from build123d import *

# Parameters (mm, degrees)
SKETCH2_W           = 8.5
SKETCH2_H           = 6
BOSS_EXTRUDE1_DEPTH = 6
SKETCH3_W           = 6
SKETCH3_H           = 12
CUT_EXTRUDE1_DEPTH  = 6


with BuildPart() as part:
    # Sketch2 → Boss-Extrude1 (new body)
    with BuildSketch(Plane.XY):
        with Locations((-58.25, 3)):
            Rectangle(SKETCH2_W, SKETCH2_H)
        Polygon((-68.5, 72), (-68.5, 0), (-62.5, 0), (-62.5, 6), (-54, 6), (-42, 6), (-42, 0), (-30, 0), (-30, 6), (-18, 6), (-18, 0), (-6, 0), (-6, 6), (6, 6), (6, 0), (18, 0), (18, 6), (30, 6), (30, 0), (42, 0), (42, 6), (54, 6), (54, 0), (68.5, 0), (68.5, 72), (54, 72), (54, 66), (42, 66), (42, 72), (30, 72), (30, 66), (18, 66), (18, 72), (6, 72), (6, 66), (-6, 66), (-6, 72), (-18, 72), (-18, 66), (-30, 66), (-30, 72), (-42, 72), (-42, 66), (-54, 66), (-54, 72), align=None)
    extrude(amount=BOSS_EXTRUDE1_DEPTH)

    # Sketch3 → Cut-Extrude1 (cut)
    with BuildSketch(Plane.XY.offset(6)):
        with Locations((-65.5, 60)):
            Rectangle(SKETCH3_W, SKETCH3_H)
        with Locations((-65.5, 12)):
            Rectangle(SKETCH3_W, SKETCH3_H)
        with Locations((65.5, 36)):
            Rectangle(SKETCH3_W, SKETCH3_H)
        with Locations((65.5, 12)):
            Rectangle(SKETCH3_W, SKETCH3_H)
        with Locations((-65.5, 36)):
            Rectangle(SKETCH3_W, SKETCH3_H)
        with Locations((65.5, 60)):
            Rectangle(SKETCH3_W, SKETCH3_H)
    extrude(amount=-CUT_EXTRUDE1_DEPTH, mode=Mode.SUBTRACT)


solid = part.part
The listing builds one solid part. Answer for the finished solid, in the listing's coordinates (mm). A direction names the side the tool comes from. Give positions to 0.01 mm unless a question says otherwise; leave off trailing zeros. Write each loop counter-clockwise with the first axis right and the second up, starting at its lowest first coordinate (ties: lowest second). Pieces come first, ordered by that corner, then holes.
Item 1: Determine the mould class of faces 5 (the flat face through (-54, 3, 3)), 6 (the flat face through (-66, 42, 3)), 7 (the flat face through (68.5, 24, 3)) for opening direction X: released by +X, released by -X, zero draft, split by the parting line, or undercut.
Item 2: Flat-ended cylindrical pins translate along their axes: P1, Ø1.8, axis at x = 22.5, z = 4, coming from the +Y side; P2, Ø1.8, axis at y = 14, z = 4, coming from the +X side. Find the tip coordinate at first contact, or state that the pin passes through.
Item 3: Find the intervals of material crossed by line 1 along X through (y, z) = (67, 0.4); line 2 along Y through (x, z) = (-21, 2.4); line 3 along X through (y, z) = (31.5, 1.25), in increasing order.
Item 4: Section B-B, the plane x = -46 is taken. Write down the section's boundary in (y, z), plus the area to 3 significant figures.
Item 5: Section A-A, the plane y = 11 is taken. Write down the section's boundary in (x, z), plus the area to 3 significant figures.
Item 6: Which of the six approach directions +Z, -Z, +X, -X, +Y, -Y give full straight-line access (tool end or side, diameter ignored) to faces 1 (the flat face through (12, 72, 3)), 2 (the flat face through (-48, 66, 3)), 3 (the flat face through (-66, 6, 3)), 4 (the flat face through (-24, 6, 3))?
Completed:
1. face 5: undercut
1. face 6: zero draft
1. face 7: released by +X
2. P1: stops at y = 66
2. P2: stops at x = 62.5
3. line 1: x = -68.5 to -54, -42 to -30, -18 to -6, 6 to 18, 30 to 42, 54 to 68.5
3. line 2: y = 6 to 66
3. line 3: x = -62.5 to 62.5
4. outline: (6, 0) - (66, 0) - (66, 6) - (6, 6) - close
4. area: 360 mm2
5. outline: (-62.5, 0) - (62.5, 0) - (62.5, 6) - (-62.5, 6) - close
5. area: 750 mm2
6. face 1: +Z, -Z, +X, -X, +Y
6. face 2: +Z, -Z, +Y
6. face 3: +Z, -Z, -X
6. face 4: +Z, -Z, -Y
